from build123d import *

# Parameters (mm, degrees)
SKETCH2_W            = 57.15
SKETCH2_H            = 6.35
BOSS_EXTRUDE1_DEPTH  = 63.5
SKETCH3_R            = 14.2875
CUT_EXTRUDE1_DEPTH   = 70.922121857
CHAMFER1_SIZE        = 6.35
M4_CLEARANCE_HOLE1_D = 4.5
M5_CLEARANCE_HOLE1_D = 5.5
FILLET1_R            = 0.762
CUT_EXTRUDE4_DEPTH   = 1.524


with BuildPart() as part:
    # Sketch2 → Boss-Extrude1 (new body)
    with BuildSketch(Plane(origin=(0, 0, 0), x_dir=(1, 0, 0), z_dir=(0, 1, 0))):
        Rectangle(SKETCH2_W, SKETCH2_H)
    extrude(amount=-BOSS_EXTRUDE1_DEPTH)

    # Sketch3 → Cut-Extrude1 (cut, through all)
    with BuildSketch(Plane.XY.offset(3.175)):
        with Locations((0, -28.8150046)):
            Circle(SKETCH3_R)
    extrude(amount=-CUT_EXTRUDE1_DEPTH, mode=Mode.SUBTRACT)

    # Chamfer1
    chamfer1_edges = [part.edges().sort_by_distance(p)[0] for p in [
        (28.575, 0, 0),
        (-28.575, 0, 0),
    ]]
    chamfer(chamfer1_edges, length=CHAMFER1_SIZE)

    # M4 Clearance Hole1 (through all)
    with Locations(Plane(origin=(0, 0, -3.175), x_dir=(-1, 0, 0), z_dir=(0, 0, -1))):
        with Locations((0.479594109, -5.08436305)):
            Hole(M4_CLEARANCE_HOLE1_D / 2)

    # M5 Clearance Hole1 (through all)
    with Locations(Plane.XY.offset(3.175)):
        with Locations((-19.05, -50.000003124), (19.05, -50.000003124)):
            Hole(M5_CLEARANCE_HOLE1_D / 2)

    # Fillet1
    fillet1_edges = [part.edges().sort_by_distance(p)[0] for p in [
        (28.575, -63.5, 0),
        (0, -63.5, -3.175),
        (0, 0, 3.175),
        (0, 0, -3.175),
        (22.225, 0, 0),
        (-22.225, 0, 0),
        (25.4, -3.175, 3.175),
        (-25.4, -3.175, 3.175),
        (-28.575, -6.35, 0),
        (25.4, -3.175, -3.175),
        (-25.4, -3.175, -3.175),
        (28.575, -6.35, 0),
        (-28.575, -63.5, 0),
        (-28.575, -34.925, -3.175),
        (28.575, -34.925, -3.175),
        (28.575, -34.925, 3.175),
        (-28.575, -34.925, 3.175),
        (0, -63.5, 3.175),
    ]]
    fillet(fillet1_edges, radius=FILLET1_R)

    # Sketch8 → Cut-Extrude4 (cut)
    with BuildSketch(Plane.XY.offset(3.175)):
        with BuildLine():
            Line((11.55, -63.5), (11.55, -49.5))
            ThreePointArc((11.55, -49.5), (19.05, -42), (26.55, -49.5))
            Line((26.55, -49.5), (26.55, -63.5))
            Line((26.55, -63.5), (11.55, -63.5))
        make_face()
    cut_extrude4 = extrude(amount=-CUT_EXTRUDE4_DEPTH, mode=Mode.SUBTRACT)

    # Mirror1: Cut-Extrude4 across plane
    add(cut_extrude4.mirror(Plane(origin=(0, 0, 0), x_dir=(0, 0, 1), z_dir=(1, 0, 0))), mode=Mode.SUBTRACT)


solid = part.part
Model file for the job. Use its own axes, mm. A direction names the side the tool comes from. Give positions to 0.01 mm unless a question says otherwise; leave off trailing zeros. Write each loop counter-clockwise with the first axis right and the second up, starting at its lowest first coordinate (ties: lowest second). Pieces come first, ordered by that corner, then holes. Notation, with made-up numbers: M 81.25,-34.5 L 115.25,-34.5 A22 cw 115.25,2.5 Z; hole C 78.5,-26.75 d2. An arc over 180 degrees is marked long. One line per item, written item: value. Start each with the question number.
Q1. Saw through at D-D, the plane x = 0. Write the cut outline in (y, z) (1 decimal), plus the area to 3 significant figures.
Q2. Drop a flat-ended pin along its axis: pin 1 Ø4.5 at (x, y) = (-17, -49) entering from +Z. Give the stop position or say it passes through.
Q3. 3-axis set-ups, long thin cutter, end or side, ignore diameter. For faces 1 (the cylindrical face through (-19, -42, 2)), 2 (the flat face through (0, -63.5, 0)): which of +Z, -Z, +X, -X, +Y, -Y reach the whole face in a straight line?
Q4. Saw through at B-B, the plane y = -22.5. Write the cut outline in (x, z) (3 decimals).
Q5. Probe probe 1 along X at (y, z) = (-50, 0) (3 decimals); probe 2 along Y at (x, z) = (19.05, -1.3); probe 3 along X at (y, z) = (-47.5, -3). List the from-to ranges inside material, lowest first. Write a range as [from, to].
Q6. Two-plate mould, pull along X, no slides. Class faces 3 (the flat face through (12, -18, 3.175)), 4 (the cylindrical face through (-25.2, -3.3, 2.96)), 5 (the cylindrical face through (-18.454, -52.685, -0.796)): +X half, -X half, draft (parallel to the pull), parting line (faces both ways), or undercut.
Q7. Saw through at C-C, the plane z = 0.5. State how many separate pieces and enclosed holes the cut face has, plus the area to 3 significant figures.
Q8. Saw through at A-A, the plane x = 19.05. Write the cut outline in (y, z) (3 decimals), plus the area to 3 significant figures.
Output values:
1. outline: M -63.5,-2.4 A0.8 ccw -62.7,-3.2 L -43.1,-3.2 L -43.1,3.2 L -62.7,3.2 A0.8 ccw -63.5,2.4 Z; M -14.5,-3.2 L -7.3,-3.2 L -7.3,3.2 L -14.5,3.2 Z; M -2.9,-3.2 L -0.8,-3.2 A0.8 ccw 0,-2.4 L 0,2.4 A0.8 ccw -0.8,3.2 L -2.9,3.2 Z
1. area: 193 mm²
2. pin 1: stops at z = 1.65
3. face 1: +Z, -Y
3. face 2: +Z, -Z, +X, -X, -Y
4. outline: M -28.575,-2.413 A0.762 ccw -27.813,-3.175 L -12.816,-3.175 L -12.816,3.175 L -27.813,3.175 A0.762 ccw -28.575,2.413 Z; M 12.816,-3.175 L 27.813,-3.175 A0.762 ccw 28.575,-2.413 L 28.575,2.413 A0.762 ccw 27.813,3.175 L 12.816,3.175 Z
5. probe 1: x = [-28.575, -21.8], [-16.3, 16.3], [21.8, 28.575]
5. probe 2: y = [-63.5, -52.75], [-47.25, 0]
5. probe 3: x = [-28.3, -20.2], [-17.9, 17.9], [20.2, 28.3]
6. face 3: draft
6. face 4: -X half
6. face 5: undercut
7. separate pieces: 1
7. enclosed holes: 4
7. area: 2,880 mm²
8. outline: M -63.5,-2.413 A0.762 ccw -62.738,-3.175 L -52.75,-3.175 L -52.75,1.651 L -63.5,1.651 Z; M -47.25,-3.175 L -0.762,-3.175 A0.762 ccw 0,-2.413 L 0,2.413 A0.762 ccw -0.762,3.175 L -42,3.175 L -42,1.651 L -47.25,1.651 Z
8. area: 344 mm²
